Work out the finished part from the listing and answer in its coordinate system (mm). Face numbers are marked on the shaded views. A direction names the side the tool comes from. Round coordinates to 2 decimals unless told otherwise and drop trailing zeros. Order: outer loops, then holes, each group sorted by start corner. A loop starts at its lowest first (then second) coordinate and runs counter-clockwise, first axis right, second up. Notation, with made-up numbers: (35, 39.5) -> (79, 39.5) arc R21 ccw to (79, 74.5) -> close; hole circle Ø1 at (45, -32.75). An arc over 180 degrees is marked (long way). Use one line per item in the form item = value.
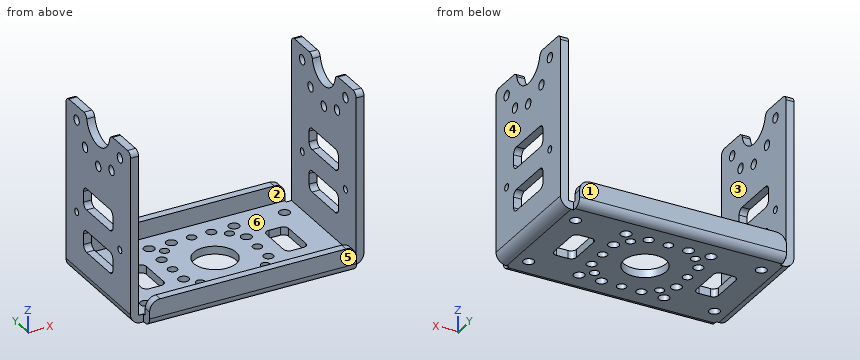
```python
from build123d import *

# Parameters (mm, degrees)
SKETCH1_W            = 39
SKETCH1_H            = 26
SKETCH1_R            = 4
SKETCH1_R_2          = 1
SKETCH1_R_3          = 0.875
SKETCH1_R_4          = 0.925
SKETCH1_R_5          = 0.85
BOSS_EXTRUDE1_DEPTH  = 1.5
SKETCH2_W            = 1.5
SKETCH2_H            = 22
BOSS_EXTRUDE2_DEPTH  = 1
SKETCH3_R            = 0.9
SKETCH3_R_2          = 0.65
BOSS_EXTRUDE3_DEPTH  = 1.5
FILLET1_R            = 2
FILLET2_R            = 1
FILLET1_OF_MIRROR1_R = 2
FILLET2_OF_MIRROR1_R = 1
SKETCH4_W            = 39
SKETCH4_H            = 4.8
BOSS_EXTRUDE4_DEPTH  = 1.5
FILLET3_R            = 2
FILLET4_R            = 1.5
SKETCH5_W            = 39
SKETCH5_H            = 4.8
BOSS_EXTRUDE5_DEPTH  = 1.5
FILLET5_R            = 2
FILLET6_R            = 1.5


with BuildPart() as part:
    # Sketch1 → Boss-Extrude1 (new body)
    with BuildSketch(Plane.XY):
        Rectangle(SKETCH1_W, SKETCH1_H)
        Circle(SKETCH1_R, mode=Mode.SUBTRACT)
        with Locations((-8, 8)):
            Circle(SKETCH1_R_2, mode=Mode.SUBTRACT)
        with Locations((-8, -8)):
            Circle(SKETCH1_R_2, mode=Mode.SUBTRACT)
        with Locations((-8, -3.8)):
            Circle(SKETCH1_R_2, mode=Mode.SUBTRACT)
        with Locations((-8, 0)):
            Circle(SKETCH1_R_3, mode=Mode.SUBTRACT)
        with Locations((-8, 3.72)):
            Circle(SKETCH1_R_4, mode=Mode.SUBTRACT)
        with Locations((8, 8)):
            Circle(SKETCH1_R_2, mode=Mode.SUBTRACT)
        with Locations((3.72, 8)):
            Circle(SKETCH1_R_4, mode=Mode.SUBTRACT)
        with Locations((0, 8)):
            Circle(SKETCH1_R_3, mode=Mode.SUBTRACT)
        with Locations((-3.8, 8)):
            Circle(SKETCH1_R_2, mode=Mode.SUBTRACT)
        with Locations((8, -8)):
            Circle(SKETCH1_R_2, mode=Mode.SUBTRACT)
        with Locations((8, -3.72)):
            Circle(SKETCH1_R_4, mode=Mode.SUBTRACT)
        with Locations((8, 0)):
            Circle(SKETCH1_R_3, mode=Mode.SUBTRACT)
        with Locations((8, 3.8)):
            Circle(SKETCH1_R_2, mode=Mode.SUBTRACT)
        with Locations((-3.72, -8)):
            Circle(SKETCH1_R_4, mode=Mode.SUBTRACT)
        with Locations((0, -8)):
            Circle(SKETCH1_R_3, mode=Mode.SUBTRACT)
        with Locations((3.8, -8)):
            Circle(SKETCH1_R_2, mode=Mode.SUBTRACT)
        with Locations((6.12616703, 6.12616703)):
            Circle(SKETCH1_R_5, mode=Mode.SUBTRACT)
        with Locations((6.12616703, -6.12616703)):
            Circle(SKETCH1_R_5, mode=Mode.SUBTRACT)
        with Locations((-6.12616703, -6.12616703)):
            Circle(SKETCH1_R_5, mode=Mode.SUBTRACT)
        with Locations((-6.12616703, 6.12616703)):
            Circle(SKETCH1_R_5, mode=Mode.SUBTRACT)
        with Locations((17.5, 8)):
            Circle(SKETCH1_R_2, mode=Mode.SUBTRACT)
        with Locations((17.5, -8)):
            Circle(SKETCH1_R_2, mode=Mode.SUBTRACT)
        with Locations((-17.5, -8)):
            Circle(SKETCH1_R_2, mode=Mode.SUBTRACT)
        with Locations((-17.5, 8)):
            Circle(SKETCH1_R_2, mode=Mode.SUBTRACT)
        with BuildLine():
            Line((12.3, 3.925), (14.5, 3.925))
            ThreePointArc((14.5, 3.925), (15.207106781, 3.632106781), (15.5, 2.925))
            Line((15.5, 2.925), (15.5, -2.925))
            ThreePointArc((15.5, -2.925), (15.207106781, -3.632106781), (14.5, -3.925))
            Line((14.5, -3.925), (12.3, -3.925))
            ThreePointArc((12.3, -3.925), (11.592893219, -3.632106781), (11.3, -2.925))
            Line((11.3, -2.925), (11.3, 2.925))
            ThreePointArc((11.3, 2.925), (11.592893219, 3.632106781), (12.3, 3.925))
        make_face(mode=Mode.SUBTRACT)
        with BuildLine():
            Line((-12.3, 3.925), (-14.5, 3.925))
            ThreePointArc((-14.5, 3.925), (-15.207106781, 3.632106781), (-15.5, 2.925))
            Line((-15.5, 2.925), (-15.5, -2.925))
            ThreePointArc((-15.5, -2.925), (-15.207106781, -3.632106781), (-14.5, -3.925))
            Line((-14.5, -3.925), (-12.3, -3.925))
            ThreePointArc((-12.3, -3.925), (-11.592893219, -3.632106781), (-11.3, -2.925))
            Line((-11.3, -2.925), (-11.3, 2.925))
            ThreePointArc((-11.3, 2.925), (-11.592893219, 3.632106781), (-12.3, 3.925))
        make_face(mode=Mode.SUBTRACT)
    extrude(amount=BOSS_EXTRUDE1_DEPTH)

    # Sketch2 → Boss-Extrude2 (add)
    with BuildSketch(Plane.ZY.offset(19.5)):
        with Locations((0.75, 0)):
            Rectangle(SKETCH2_W, SKETCH2_H)
    boss_extrude2 = extrude(amount=BOSS_EXTRUDE2_DEPTH)

    # Sketch3 → Boss-Extrude3 (add)
    with BuildSketch(Plane.ZY.offset(20.5)):
        with BuildLine():
            Line((0, 11), (32.5, 11))
            Line((32.5, 11), (32.5, 4))
            ThreePointArc((32.5, 4), (28.5, 0), (32.5, -4))
            Line((32.5, -4), (32.5, -11))
            Line((32.5, -11), (0, -11))
            Line((0, -11), (0, 11))
        make_face()
        with Locations((24.65, 0)):
            Circle(SKETCH3_R, mode=Mode.SUBTRACT)
        with Locations((26.069656452, 4.502575025)):
            Circle(SKETCH3_R, mode=Mode.SUBTRACT)
        with Locations((29.815141875, 7.376587073)):
            Circle(SKETCH3_R, mode=Mode.SUBTRACT)
        with Locations((29.815141875, -7.376587073)):
            Circle(SKETCH3_R, mode=Mode.SUBTRACT)
        with Locations((26.069656452, -4.502575025)):
            Circle(SKETCH3_R, mode=Mode.SUBTRACT)
        with Locations((12.5, 7.376587073)):
            Circle(SKETCH3_R_2, mode=Mode.SUBTRACT)
        with Locations((12.5, -7.376587073)):
            Circle(SKETCH3_R_2, mode=Mode.SUBTRACT)
        with BuildLine():
            Line((15.5, -5), (17.5, -5))
            ThreePointArc((17.5, -5), (18.207106781, -4.707106781), (18.5, -4))
            Line((18.5, -4), (18.5, 4))
            ThreePointArc((18.5, 4), (18.207106781, 4.707106781), (17.5, 5))
            Line((17.5, 5), (15.5, 5))
            ThreePointArc((15.5, 5), (14.792893219, 4.707106781), (14.5, 4))
            Line((14.5, 4), (14.5, -4))
            ThreePointArc((14.5, -4), (14.792893219, -4.707106781), (15.5, -5))
        make_face(mode=Mode.SUBTRACT)
        with BuildLine():
            Line((7.5, 5), (9.5, 5))
            ThreePointArc((9.5, 5), (10.207106781, 4.707106781), (10.5, 4))
            Line((10.5, 4), (10.5, -4))
            ThreePointArc((10.5, -4), (10.207106781, -4.707106781), (9.5, -5))
            Line((9.5, -5), (7.5, -5))
            ThreePointArc((7.5, -5), (6.792893219, -4.707106781), (6.5, -4))
            Line((6.5, -4), (6.5, 4))
            ThreePointArc((6.5, 4), (6.792893219, 4.707106781), (7.5, 5))
        make_face(mode=Mode.SUBTRACT)
    boss_extrude3 = extrude(amount=BOSS_EXTRUDE3_DEPTH)

    # Fillet1
    fillet1_edges = [part.edges().sort_by_distance(p)[0] for p in [
        (-22, 0, 0),
    ]]
    fillet(fillet1_edges, radius=FILLET1_R)

    # Fillet2
    fillet2_edges = [part.edges().sort_by_distance(p)[0] for p in [
        (-21.25, 11, 32.5),
        (-21.25, 4, 32.5),
        (-21.25, -4, 32.5),
        (-21.25, -11, 32.5),
    ]]
    fillet(fillet2_edges, radius=FILLET2_R)

    # Mirror1: Boss-Extrude2, Boss-Extrude3 across plane
    add(boss_extrude2.mirror(Plane(origin=(0, 0, 0), x_dir=(0, 0, 1), z_dir=(1, 0, 0))))
    add(boss_extrude3.mirror(Plane(origin=(0, 0, 0), x_dir=(0, 0, 1), z_dir=(1, 0, 0))))

    # Fillet1 of Mirror1
    fillet1_of_mirror1_edges = [part.edges().sort_by_distance(p)[0] for p in [
        (22, 0, 0),
    ]]
    fillet(fillet1_of_mirror1_edges, radius=FILLET1_OF_MIRROR1_R)

    # Fillet2 of Mirror1
    fillet2_of_mirror1_edges = [part.edges().sort_by_distance(p)[0] for p in [
        (21.25, 11, 32.5),
        (21.25, 4, 32.5),
        (21.25, -4, 32.5),
        (21.25, -11, 32.5),
    ]]
    fillet(fillet2_of_mirror1_edges, radius=FILLET2_OF_MIRROR1_R)

    # Sketch4 → Boss-Extrude4 (add)
    with BuildSketch(Plane(origin=(0, 13, 0), x_dir=(1, 0, 0), z_dir=(0, 1, 0))):
        with Locations((0, -2.4)):
            Rectangle(SKETCH4_W, SKETCH4_H)
    extrude(amount=-BOSS_EXTRUDE4_DEPTH)

    # Fillet3
    fillet3_edges = [part.edges().sort_by_distance(p)[0] for p in [
        (-19.5, 12.25, 4.8),
        (19.5, 12.25, 4.8),
    ]]
    fillet(fillet3_edges, radius=FILLET3_R)

    # Fillet4
    fillet4_edges = [part.edges().sort_by_distance(p)[0] for p in [
        (0, 13, 0),
    ]]
    fillet(fillet4_edges, radius=FILLET4_R)

    # Sketch5 → Boss-Extrude5 (add)
    with BuildSketch(Plane.XZ.offset(13)):
        with Locations((0, 2.4)):
            Rectangle(SKETCH5_W, SKETCH5_H)
    extrude(amount=-BOSS_EXTRUDE5_DEPTH)

    # Fillet5
    fillet5_edges = [part.edges().sort_by_distance(p)[0] for p in [
        (-19.5, -12.25, 4.8),
        (19.5, -12.25, 4.8),
    ]]
    fillet(fillet5_edges, radius=FILLET5_R)

    # Fillet6
    fillet6_edges = [part.edges().sort_by_distance(p)[0] for p in [
        (0, -13, 0),
    ]]
    fillet(fillet6_edges, radius=FILLET6_R)


solid = part.part
```
Item 1: The part is cut by section C-C, the plane z = 12.5. Give the vertices of the cut face in (x, y).
Findings:
outline = (-22, -11) -> (-20.5, -11) -> (-20.5, -8.03) -> (-22, -8.03) -> close; (-22, -6.73) -> (-20.5, -6.73) -> (-20.5, 6.73) -> (-22, 6.73) -> close; (-22, 8.03) -> (-20.5, 8.03) -> (-20.5, 11) -> (-22, 11) -> close; (20.5, -11) -> (22, -11) -> (22, -8.03) -> (20.5, -8.03) -> close; (20.5, -6.73) -> (22, -6.73) -> (22, 6.73) -> (20.5, 6.73) -> close; (20.5, 8.03) -> (22, 8.03) -> (22, 11) -> (20.5, 11) -> close
Item 2: For the marked faces 1, 2 and 3, determine the directions among +Z, -Z, +X, -X, +Y, -Y from which every point of the face is accessible in a straight line to the end or side of a thin tool.
Findings:
face_1 = +Z, -Z, +X, -X, +Y
face_2 = +Z, +X, -X
face_3 = +Z, +Y, -Y
Item 3: The part is cut by section B-B, the plane z = 8.5. Give the vertices of the cut face in (x, y), and give its area (3 significant figures).
Findings:
outline = (-22, -11) -> (-20.5, -11) -> (-20.5, -5) -> (-22, -5) -> close; (-22, 5) -> (-20.5, 5) -> (-20.5, 11) -> (-22, 11) -> close; (20.5, -11) -> (22, -11) -> (22, -5) -> (20.5, -5) -> close; (20.5, 5) -> (22, 5) -> (22, 11) -> (20.5, 11) -> close
area = 36.0 mm^2
Item 4: Consider line 1 along X through (y, z) = (8.5, 21); line 2 along Y through (x, z) = (-21, 12); line 3 along Y through (x, z) = (17, 1). Determine where each line is inside the solid, lowest interval first.
Findings:
line_1 = -22 to -20.5, 20.5 to 22
line_2 = -11 to -7.79, -6.96 to 6.96, 7.79 to 11
line_3 = -12.91 to -8.87, -7.13 to 7.13, 8.87 to 12.91
Item 5: The part is cut by section D-D, the plane x = 0. Give the vertices of the cut face in (y, z) (3 decimals).
Findings:
outline = (-13, 1.5) arc R1.5 ccw to (-11.5, 0) -> (-8.875, 0) -> (-8.875, 1.5) -> (-11.5, 1.5) -> (-11.5, 4.8) -> (-13, 4.8) -> close; (-7.125, 0) -> (-4, 0) -> (-4, 1.5) -> (-7.125, 1.5) -> close; (4, 0) -> (7.125, 0) -> (7.125, 1.5) -> (4, 1.5) -> close; (8.875, 0) -> (11.5, 0) arc R1.5 ccw to (13, 1.5) -> (13, 4.8) -> (11.5, 4.8) -> (11.5, 1.5) -> (8.875, 1.5) -> close
Item 6: The part is cut by section A-A, the plane x = -14. Give the vertices of the cut face in (y, z) (3 decimals).
Findings:
outline = (-13, 1.5) arc R1.5 ccw to (-11.5, 0) -> (-3.925, 0) -> (-3.925, 1.5) -> (-11.5, 1.5) -> (-11.5, 4.8) -> (-13, 4.8) -> close; (3.925, 0) -> (11.5, 0) arc R1.5 ccw to (13, 1.5) -> (13, 4.8) -> (11.5, 4.8) -> (11.5, 1.5) -> (3.925, 1.5) -> close
Item 7: Determine the mould class of the marked faces 4, 5 and 6 for opening direction X: released by +X, released by -X, zero draft, split by the parting line, or undercut.
Findings:
face_4 = released by +X
face_5 = zero draft
face_6 = undercut
Item 8: Flat-ended cylindrical pins translate along their axes: P1, Ø5, axis at x = 9, z = 9, coming from the +Y side; P2, Ø6, axis at x = 2.5, y = -9, coming from the +Z side; P3, Ø3, axis at x = 8, y = -3.72, coming from the +Z side; P4, Ø0.8, axis at x = 21, y = -0.5, coming from the +Z side. Find the tip coordinate at first contact, or state that the pin passes through.
Findings:
P1 = through
P2 = 4.8
P3 = 1.5
P4 = 28.6
